Here's the drawing with two shaded views (mm, measured from the low corner). I have some questions. A direction names the side the tool comes from. Round coordinates to 2 decimals unless told otherwise and drop trailing zeros. Write each loop counter-clockwise with the first axis right and the second up, starting at its lowest first coordinate (ties: lowest second). Pieces come first, ordered by that corner, then holes. Notation, with made-up numbers: M -2.5,39.25 L 14.5,39.25 A22 cw 14.5,61.25 Z; hole C 22,55 d3. An arc over 180 degrees is marked long. Use one line per item in the form item = value. Start each with the question number.
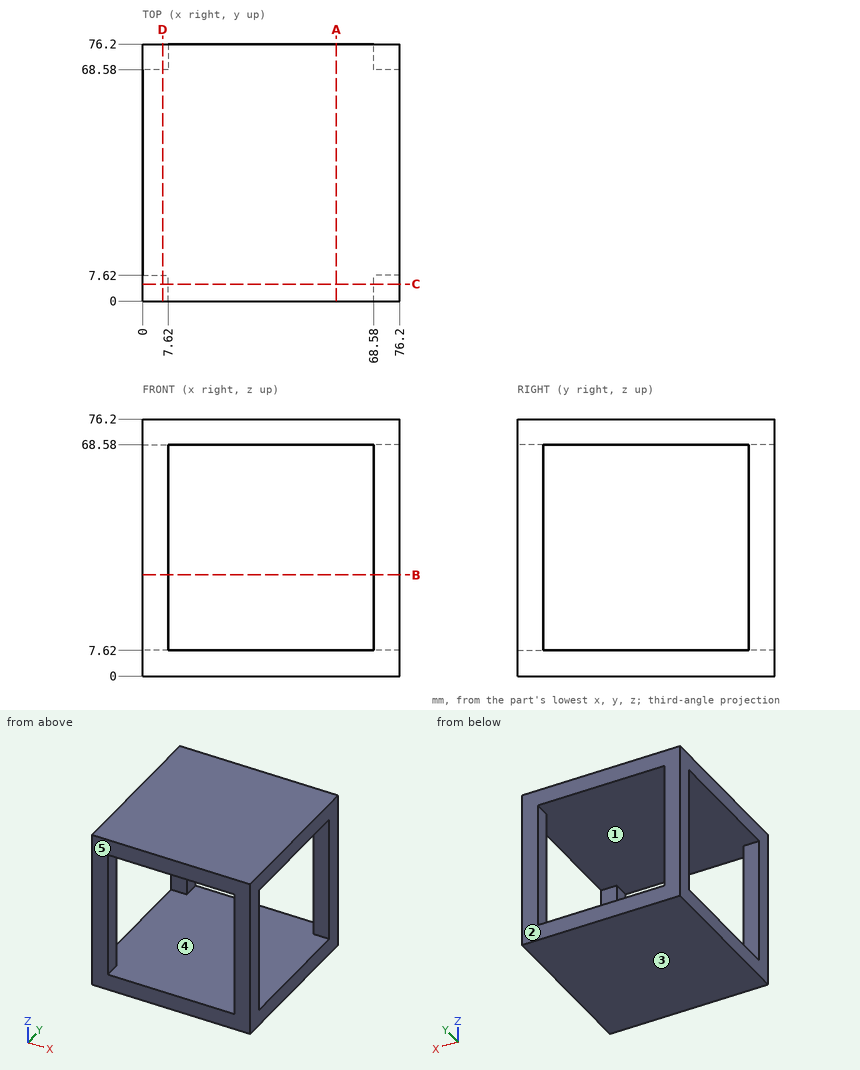
1. Please list where this line runs through material, in increasing order: line 1 along Z through (x, y) = (21, 62).
2. If we mould it in two halves opening along Y, with no side actions, what happens to the marked faces 3, 4 and 5? For each: pulls with the +Y half, pulls with the -Y half, needs draft (parallel to the pull), parting line crosses it, or undercut.
3. If we section it at C-C (y = 5): List the corners of the cut face in (x, z) for me.
4. Which directions (+Z, -Z, +X, -X, +Y, -Y) give clear straight access to the entire face, cutting with the end or side of a thin tool? Please do the marked faces 1 and 2.
5. If we section it at B-B (z = 30): List the corners of the cut face in (x, y) for me.
6. If we section it at A-A (x = 57.5): List the corners of the cut face in (y, z) for me.
Model answer:
q1.line_1 = 0 to 7.62, 68.58 to 76.2
q2.face_3 = needs draft
q2.face_4 = undercut
q2.face_5 = pulls with the -Y half
q3.outline = M 0,0 L 76.2,0 L 76.2,76.2 L 0,76.2 Z; hole M 7.62,7.62 L 68.58,7.62 L 68.58,68.58 L 7.62,68.58 Z
q4.face_1 = none
q4.face_2 = +Z, -Z, +X, -X, +Y
q5.outline = M 0,0 L 7.62,0 L 7.62,7.62 L 0,7.62 Z; M 0,68.58 L 7.62,68.58 L 7.62,76.2 L 0,76.2 Z; M 68.58,0 L 76.2,0 L 76.2,7.62 L 68.58,7.62 Z; M 68.58,68.58 L 76.2,68.58 L 76.2,76.2 L 68.58,76.2 Z
q6.outline = M 0,0 L 76.2,0 L 76.2,7.62 L 0,7.62 Z; M 0,68.58 L 76.2,68.58 L 76.2,76.2 L 0,76.2 Z
